Autodesk Inventor part; units mm, degrees
ref_plane "YZ Plane" through (0, 0, 0) normal (1, 0, 0) x (0, 1, 0)
ref_plane "XZ Plane" through (0, 0, 0) normal (0, 1, 0) x (-1, 0, 0)
ref_plane "XY Plane" through (0, 0, 0) normal (0, 0, 1) x (1, 0, 0)
sketch "Эскиз1" plane through (0, 0, 0) normal (0, 0, 1) x (1, 0, 0)
  line L0 (0, 0) -> (64.3, 0)
  line L1 (64.3, 0) -> (64.3, -50.7)
  line L2 (64.3, -50.7) -> (0, -50.7)
  line L3 (0, -50.7) -> (0, 0)
  dimension "d0" = 64.3
  dimension "d1" = 50.7
extrude "Выдавливание1" add sketch "Эскиз1" along normal blind 7.6
sketch "Эскиз2" plane through (0, -50.7, 0) normal (0, -1, 0) x (1, 0, 0)
  line L0 (0, 0) -> (64.3, 0)
  line L1 (0, 0) -> (32.15, 0)
  line L2 (32.15, 0) -> (33.95, 0)
  line L3 (33.95, 0) -> (35.75, 3.1177)
  line L4 (35.75, 3.1177) -> (33.95, 6.2354)
  line L5 (33.95, 6.2354) -> (30.35, 6.2354)
  line L6 (30.35, 6.2354) -> (28.55, 3.1177)
  line L7 (28.55, 3.1177) -> (30.35, 0)
  line L8 (30.35, 0) -> (32.15, 0)
  dimension "d4" = 32.15
  dimension "d5" = 1.8
  dimension "d6" = 3.6
  dimension "d7" = 120
  dimension "d8" = 3.6
  dimension "d9" = 120
extrude "Выдавливание2" cut sketch "Эскиз2" against normal blind 3.8
sketch "Эскиз3" plane through (0, -50.7, 7.6) normal (0, -1, 0) x (1, 0, 0)
  circle A0 centre (32.15, -4.4823) radius 1.8
  point P0 (0, -7.6)
  dimension "d12" = 3.6
extrude "Выдавливание3" cut sketch "Эскиз3" against normal blind 6.8
sketch "Эскиз4" plane through (0, -50.7, 7.6) normal (0, -1, 0) x (1, 0, 0)
  circle A0 centre (32.15, -4.4823) radius 1.8
  line L0 (32.15, -4.4823) -> (37.65, -4.4823)
  line L1 (64.3, -7.6) -> (33.95, -7.6)
  line L2 (0, 0) -> (64.3, 0)
  line L3 (37.65, -7.6) -> (26.65, -7.6)
  line L4 (26.65, -7.6) -> (26.65, 0)
  line L5 (26.65, 0) -> (37.65, 0)
  line L6 (37.65, 0) -> (37.65, -7.6)
  point P0 (0, -7.6)
  dimension "d15" = 5.5
  dimension "d16" = 11
extrude "Выдавливание4" cut sketch "Эскиз4" against normal blind 1
fillet "Сопряжение1" radius 9 2 edges at (0, 0, 3.8) (64.3, 0, 3.8)
sketch "Эскиз5" plane through (0, 0, 7.6) normal (0, 0, 1) x (1, 0, 0)
  line L0 (0, 0) -> (8.864, -0.001)
  arc A0 (9, 0) -> (0, -9) centre (9, -9) ccw
  line L1 (8.864, -0.001) -> (8.863, -8.865)
  circle A1 centre (8.863, -8.865) radius 1.8
  line L2 (64.3, 0) -> (55.436, 0)
  line L3 (55.3, 0) -> (9, 0)
  line L4 (55.436, 0) -> (55.436, -8.864)
  circle A2 centre (55.436, -8.864) radius 1.8
  dimension "d20" = 8.864
  dimension "d21" = 8.864
  dimension "d22" = 3.6
  dimension "d23" = 8.864
  dimension "d24" = 8.864
  dimension "d25" = 90
  dimension "d26" = 3.6
extrude "Выдавливание5" cut sketch "Эскиз5" against normal blind 10
sketch "Эскиз6" plane through (0, 0, 7.6) normal (0, 0, 1) x (1, 0, 0)
  circle A0 centre (8.863, -8.865) radius 1.8
  line L0 (8.863, -8.865) -> (8.863, -42.636)
  circle A1 centre (8.863, -42.636) radius 1.8
  circle A2 centre (55.436, -8.864) radius 1.8
  line L1 (55.436, -8.864) -> (55.436, -42.635)
  circle A3 centre (55.436, -42.635) radius 1.8
  point P0 (0, 0)
  dimension "d29" = 33.771
  dimension "d30" = 3.6
  dimension "d31" = 33.771
  dimension "d32" = 3.6
extrude "Выдавливание6" cut sketch "Эскиз6" against normal blind 10 contours A1 | A3
sketch "Эскиз7" plane through (0, 0, 7.6) normal (0, 0, 1) x (1, 0, 0)
  point P0 (0, 0)
sketch "Эскиз8" plane through (0, 0, 7.6) normal (0, 0, 1) x (1, 0, 0)
  circle A0 centre (8.863, -8.865) radius 1.8
  circle A1 centre (8.863, -8.865) radius 3.55
  circle A2 centre (55.436, -8.864) radius 1.8
  circle A3 centre (55.436, -8.864) radius 3.55
  circle A4 centre (55.436, -42.635) radius 1.8
  circle A5 centre (55.436, -42.635) radius 3.55
  circle A6 centre (8.863, -42.636) radius 1.8
  circle A7 centre (8.863, -42.636) radius 3.55
  point P0 (0, 0)
  dimension "d35" = 7.1
  dimension "d36" = 7.1
  dimension "d37" = 7.1
  dimension "d38" = 7.1
extrude "Выдавливание7" cut sketch "Эскиз8" against normal blind 2.8
fillet "Сопряжение2" radius 5.5 5 edges at (2.636, -2.636, 7.6) (32.15, 0, 7.6) (61.664, -2.636, 7.6) (64.3, -29.85, 7.6) (0, -29.85, 7.6)
sketch "Эскиз9" plane through (0, 0, 0) normal (0, 0, -1) x (-1, 0, 0)
  line L0 (0, -50.7) -> (0, -9)
  line L1 (0, -50.7) -> (-31.3, -50.7)
  line L2 (-26.65, -50.7) -> (0, -50.7)
  point P0 (0, 0)
  dimension "d42" = 31.3
sketch "Эскиз10" plane through (37.65, -50.7, 0) normal (0, -1, 0) x (1, 0, 0)
  point P0 (-37.65, 0)
sketch "Эскиз11" plane through (0, -49.7, 7.6) normal (0, -1, 0) x (1, 0, 0)
  line L0 (9, -7.6) -> (55.3, -7.6)
  line L1 (36.8968, -7.6) -> (28.1351, -7.6)
  line L2 (28.1351, -7.6) -> (28.1351, -0.8108)
  line L3 (28.1351, -0.8108) -> (36.8968, -0.8108)
  line L4 (36.8968, -0.8108) -> (36.8968, -7.6)
  point P0 (0, -7.6)
extrude "Выдавливание8" add sketch "Эскиз11" against normal blind 6.8
sketch "Эскиз12" plane through (37.65, -50.7, 0) normal (0, -1, 0) x (1, 0, 0)
  line L0 (0, 7.6) -> (0, 0)
  line L1 (26.65, 0) -> (0, 0)
  line L2 (0, 7.6) -> (6, 7.6)
  line L3 (6, 7.6) -> (6, 0)
  line L4 (6, 0) -> (0, 0)
  line L5 (0, 0) -> (0, 7.6)
  point P0 (-37.65, 0)
  dimension "d45" = 6
extrude "Выдавливание9" cut sketch "Эскиз12" against normal blind 1
sketch "Эскиз13" plane through (0, -49.7, 7.6) normal (0, -1, 0) x (1, 0, 0)
  line L0 (26.65, -7.6) -> (0, -7.6)
  line L1 (0, -7.6) -> (31.3, -7.6)
  line L2 (31.3, -7.6) -> (33.1, -7.6)
  line L3 (9, -7.6) -> (55.3, -7.6)
  line L4 (43.65, 0) -> (43.65, -7.6)
  line L5 (64.3, -7.6) -> (43.65, -7.6)
  line L6 (43.65, 0) -> (47.65, 0)
  line L7 (47.65, 0) -> (47.65, -7.6)
  line L8 (47.65, -7.6) -> (43.65, -7.6)
  line L9 (43.65, -7.6) -> (43.65, 0)
  dimension "d48" = 31.3
  dimension "d49" = 1.8
  dimension "d50" = 4
extrude "Выдавливание10" cut sketch "Эскиз13" along normal blind 1
sketch "Эскиз14" plane through (0, -49.7, 7.6) normal (0, -1, 0) x (1, 0, 0)
  line L0 (0, -7.6) -> (37.3, -7.6)
  line L1 (9, -7.6) -> (55.3, -7.6)
  line L2 (37.3, -7.6) -> (39.1, -7.6)
  line L3 (39.1, -7.6) -> (42.7, -7.6)
  line L4 (42.7, -7.6) -> (44.5, -4.4823)
  line L5 (44.5, -4.4823) -> (42.7, -1.3646)
  line L6 (42.7, -1.3646) -> (39.1, -1.3646)
  line L7 (39.1, -1.3646) -> (37.3, -4.4823)
  line L8 (37.3, -4.4823) -> (39.1, -7.6)
  dimension "d53" = 37.3
  dimension "d54" = 1.8
  dimension "d55" = 3.6
  dimension "d56" = 3.6
  dimension "d57" = 120
  dimension "d58" = 3.6
  dimension "d59" = 120
extrude "Выдавливание11" cut sketch "Эскиз14" against normal blind 2.8
sketch "Эскиз15" plane through (0, -49.7, 7.6) normal (0, -1, 0) x (1, 0, 0)
  circle A0 centre (40.9, -4.4823) radius 1.8
  point P0 (0, -7.6)
  dimension "d62" = 3.6
extrude "Выдавливание12" cut sketch "Эскиз15" against normal blind 6.8
sketch "Эскиз16" plane through (0, -49.7, 7.6) normal (0, -1, 0) x (1, 0, 0)
  circle A0 centre (40.9, -4.4823) radius 1.8
  line L0 (40.9, -4.4823) -> (46.4, -4.4823)
  line L1 (47.65, -7.6) -> (47.65, 0)
  line L2 (46.4, -7.6) -> (47.65, -7.6)
  line L3 (47.65, -7.6) -> (47.65, 0)
  line L4 (47.65, 0) -> (46.4, 0)
  line L5 (46.4, 0) -> (46.4, -7.6)
  point P0 (0, -7.6)
  dimension "d65" = 5.5
extrude "Выдавливание13" add sketch "Эскиз16" along normal blind 1 contours L5 L4 L1 L2
sketch "Эскиз17" plane through (0, -49.7, 7.6) normal (0, -1, 0) x (1, 0, 0)
  circle A0 centre (40.9, -4.4823) radius 1.8
  line L0 (40.9, -4.4823) -> (46.4, -4.4823)
  line L1 (46.4, 0) -> (46.4, -7.6)
  line L2 (40.9, -4.4823) -> (35.4, -4.4823)
  line L3 (26.65, -7.6) -> (26.65, 0)
  line L4 (26.65, 0) -> (35.4, 0)
  line L5 (35.4, 0) -> (35.4, -7.6)
  line L6 (35.4, -7.6) -> (26.65, -7.6)
  line L7 (26.65, -7.6) -> (26.65, 0)
  point P0 (0, -7.6)
  dimension "d68" = 5.5
  dimension "d69" = 5.5
extrude "Выдавливание14" add sketch "Эскиз17" along normal blind 1 contours L5 L6 L3 L4
sketch "Эскиз18" plane through (0, 0, 0) normal (0, 0, -1) x (-1, 0, 0)
  line L0 (0, -50.7) -> (-38, -50.7)
  point P0 (0, 0)
  dimension "d72" = 38
sketch "Эскиз19" plane through (0, 0, 0) normal (0, 0, -1) x (-1, 0, 0)
  line L0 (0, -50.7) -> (-38, -50.7)
  line L1 (-38, -50.7) -> (-24.6, -50.7)
  line L2 (-24.6, -50.7) -> (-24.6, -48.7)
  line L3 (-24.6, -48.7) -> (-38, -48.7)
  line L4 (-38, -48.7) -> (-38, -50.7)
  point P0 (0, 0)
  dimension "d73" = 38
  dimension "d74" = 13.4
  dimension "d75" = 2
extrude "Выдавливание15" cut sketch "Эскиз19" against normal blind 1.2
properties part number "golova 3 krushka"
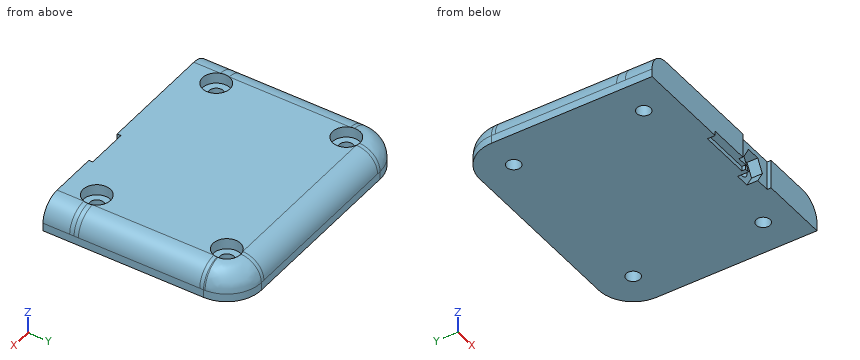
CAD build for the part. Positions are in the model's coordinates, mm. Coordinates: 2 decimals unless noted, no trailing zeros. Write each loop counter-clockwise with the first axis right and the second up, starting at its lowest first coordinate (ties: lowest second). Pieces come first, ordered by that corner, then holes. Notation, with made-up numbers: (57.25, 83.25) - (75.25, 83.25) arc R19 ccw to (75.25, 108.25) - close; hole circle Ø7 at (61, 60.5). An arc over 180 degrees is marked (long way). Use a Markdown table: item, result. Add a question column.
Item 1: Flat gauge pins, fed straight in: pin 1 (5.5 mm diameter, centred on x = 9.5, y = -42.5, fed in from +Z); pin 2 (3 mm diameter, centred on x = 41.5, z = 3, fed in from -Y); pin 3 (0.8 mm diameter, centred on y = -50, z = 3.5, fed in from -X). Where does each tip first touch, or does it go through?
Item 2: Band-saw the part on C-C, the plane z = 4. Give the number of separate pieces and of enclosed holes in the cut face, and give its area (3 significant figures).
Item 3: Band-saw the part on A-A, the plane x = 40.9. Give the cut face in (y, z), and give its area (3 significant figures).
Item 4: Drill centre lines: L1, parallel to Z at x = 40.9, y = -45.95; L2, parallel to Y at x = 58, z = 5; L3, parallel to X at y = -42, z = 1.5. Where is each one in solid material? Low to high. Write a range as from..to.
Item 5: Band-saw the part on B-B, the plane y = -23. Give the cut face in (x, z).
Numbers:
| question | item | result |
|---|---|---|
| 1 | pin 1 | z = 4.8 |
| 1 | pin 2 | y = -46.9 |
| 1 | pin 3 | x = 0.09 |
| 2 | separate pieces | 1 |
| 2 | enclosed holes | 4 |
| 2 | area | 3,090 mm2 |
| 3 | outline | (-49.7, 6.24) - (-46.9, 6.24) - (-46.9, 4.92) - (-42.9, 4.92) - (-42.9, 1.32) - (-46.9, 1.32) - (-46.9, 0) - (0, 0) - (0, 2.1) arc R5.5 ccw to (-5.5, 7.6) - (-49.7, 7.6) - close |
| 3 | area | 339 mm2 |
| 4 | L1 | 0..1.32, 4.92..7.6 |
| 4 | L2 | -50.7..-45.09, -40.18..-11.32, -6.41..-1.28 |
| 4 | L3 | 0..7.18, 10.55..53.75, 57.12..64.3 |
| 5 | outline | (0, 0) - (64.3, 0) - (64.3, 2.1) arc R5.5 ccw to (58.8, 7.6) - (5.5, 7.6) arc R5.5 ccw to (0, 2.1) - close |
